Check sheet for the drawn part. Datum: minimum x, y, z corner. Units: mm. Give positions to 0.01 mm unless a question says otherwise; leave off trailing zeros. Write each loop counter-clockwise with the first axis right and the second up, starting at its lowest first coordinate (ties: lowest second). Pieces come first, ordered by that corner, then holes. Notation, with made-up numbers: M -6,-14.5 L 8,-14.5 A25 ccw 8,10.5 Z; hole C -39,20 d6. An arc over 180 degrees is marked long. Write item = value, one per line. Start each with the question number.
1) Sectioned sample at A-A, the plane z = 50. Record the cut outline in (x, y).
2) Sectioned sample at B-B, the plane y = 5. Count the separate pieces of the cut face and the enclosed holes in it, then the cut area to 3 significant figures.
3) Scan lines: L1, parallel to X at y = 1.5, z = 42; L2, parallel to X at y = 2.5, z = 50; L3, parallel to X at y = 2.25, z = 69 (1 decimal). Record each from-to range of solid material in increasing order.
4) Sectioned sample at C-C, the plane x = 103.75. Record the cut outline in (y, z).
5) Gauge pin test, flat ends, axial feed: pin 1 (3.5 mm diameter, centred on x = 75, z = 42, fed in from +Y); pin 2 (1.9 mm diameter, centred on x = 110, z = 42, fed in from +Y). Record the tip position at first contact, or that the pin passes through.
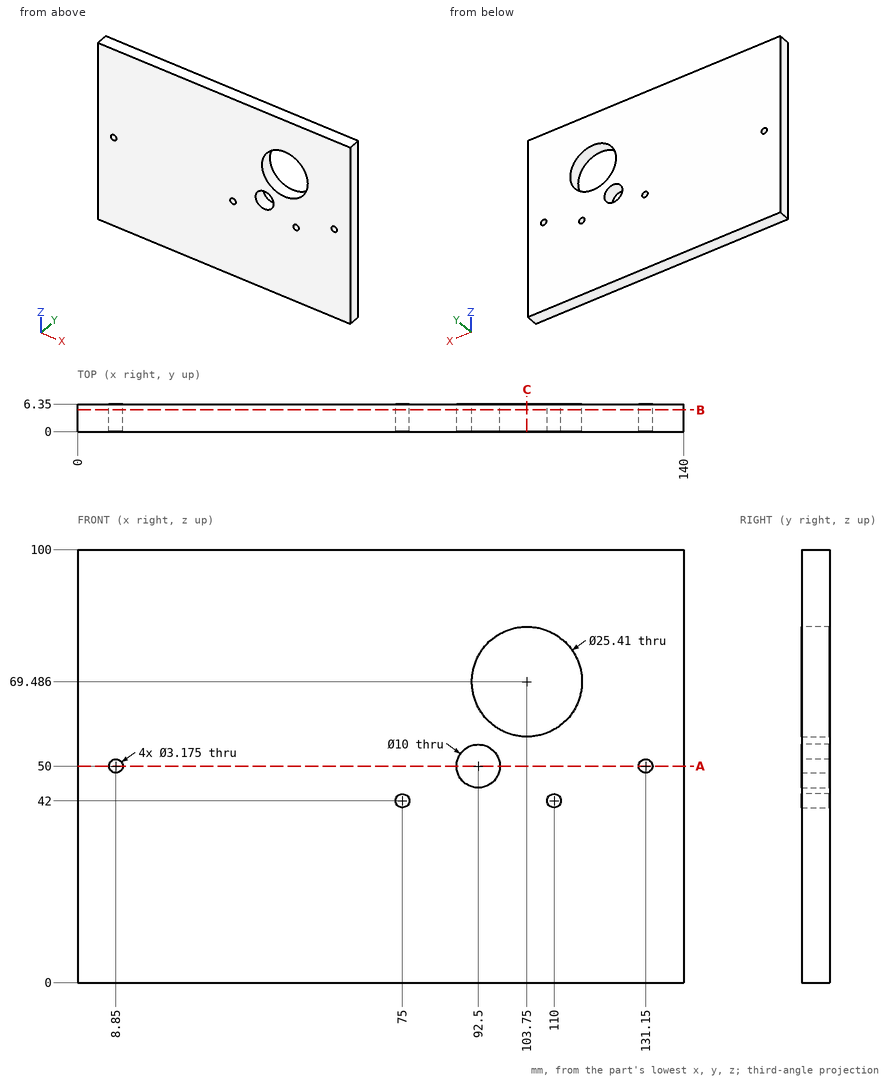
Data:
q1.outline = M 0,0 L 7.26,0 L 7.26,6.35 L 0,6.35 Z; M 10.44,0 L 87.5,0 L 87.5,6.35 L 10.44,6.35 Z; M 97.5,0 L 129.56,0 L 129.56,6.35 L 97.5,6.35 Z; M 132.74,0 L 140,0 L 140,6.35 L 132.74,6.35 Z
q2.separate_pieces = 1
q2.enclosed_holes = 6
q2.area = 13,400 mm2
q3.L1 = 0 to 73.41, 76.59 to 108.41, 111.59 to 140
q3.L2 = 0 to 7.26, 10.44 to 87.5, 97.5 to 129.56, 132.74 to 140
q3.L3 = 0 to 91.1, 116.4 to 140
q4.outline = M 0,0 L 6.35,0 L 6.35,56.78 L 0,56.78 Z; M 0,82.19 L 6.35,82.19 L 6.35,100 L 0,100 Z
q5.pin_1 = 6.35
q5.pin_2 = through
